```python
from build123d import *

# Parameters (mm, degrees)
SKETCH1_R           = 3.175
BOSS_EXTRUDE1_DEPTH = 20.6
SKETCH2_R           = 19.05
BOSS_EXTRUDE2_DEPTH = 1.6
BOSS_EXTRUDE3_DEPTH = 4.8
BOSS_EXTRUDE4_DEPTH = 51.2
SKETCH7_W           = 3.420526276
SKETCH7_H           = 1.112659396
CUT_EXTRUDE5_DEPTH  = 15
CUT_EXTRUDE6_REACH  = 58
SKETCH8_R           = 2.55
CUT_EXTRUDE7_DEPTH  = 17


with BuildPart() as part:
    # Sketch1 → Boss-Extrude1 (new body)
    with BuildSketch(Plane.XY):
        Circle(SKETCH1_R)
    extrude(amount=BOSS_EXTRUDE1_DEPTH)

    # Sketch2 → Boss-Extrude2 (add)
    with BuildSketch(Plane(origin=(0, 0, 0), x_dir=(-1, 0, 0), z_dir=(0, 0, -1))):
        Circle(SKETCH2_R)
    extrude(amount=-BOSS_EXTRUDE2_DEPTH)

    # Sketch3 → Boss-Extrude3 (add)
    with BuildSketch(Plane(origin=(0, 0, 0), x_dir=(-1, 0, 0), z_dir=(0, 0, -1))):
        with BuildLine():
            Line((23.6, -28.2), (-23.6, -28.2))
            ThreePointArc((-23.6, -28.2), (-26.852691193, -26.852691193), (-28.2, -23.6))
            Line((-28.2, -23.6), (-28.2, 23.6))
            ThreePointArc((-28.2, 23.6), (-26.852691193, 26.852691193), (-23.6, 28.2))
            Line((-23.6, 28.2), (23.6, 28.2))
            ThreePointArc((23.6, 28.2), (26.852691193, 26.852691193), (28.2, 23.6))
            Line((28.2, 23.6), (28.2, -23.6))
            ThreePointArc((28.2, -23.6), (26.852691193, -26.852691193), (23.6, -28.2))
        make_face()
    extrude(amount=BOSS_EXTRUDE3_DEPTH)

    # Sketch4 → Boss-Extrude4 (add)
    with BuildSketch(Plane(origin=(0, 0, -4.8), x_dir=(-1, 0, 0), z_dir=(0, 0, -1))):
        with BuildLine():
            Line((-18.57, 23.57), (-18.57, 25.7))
            ThreePointArc((-18.57, 25.7), (-17.837766953, 27.467766953), (-16.07, 28.2))
            Line((-16.07, 28.2), (16.07, 28.2))
            ThreePointArc((16.07, 28.2), (17.837766953, 27.467766953), (18.57, 25.7))
            Line((18.57, 25.7), (18.57, 23.57))
            ThreePointArc((18.57, 23.57), (20.034466094, 20.034466094), (23.57, 18.57))
            Line((23.57, 18.57), (25.7, 18.57))
            ThreePointArc((25.7, 18.57), (27.467766953, 17.837766953), (28.2, 16.07))
            Line((28.2, 16.07), (28.2, -16.07))
            ThreePointArc((28.2, -16.07), (27.467766953, -17.837766953), (25.7, -18.57))
            Line((25.7, -18.57), (23.57, -18.57))
            ThreePointArc((23.57, -18.57), (20.034466094, -20.034466094), (18.57, -23.57))
            Line((18.57, -23.57), (18.57, -25.7))
            ThreePointArc((18.57, -25.7), (17.837766953, -27.467766953), (16.07, -28.2))
            Line((16.07, -28.2), (-16.07, -28.2))
            ThreePointArc((-16.07, -28.2), (-17.837766953, -27.467766953), (-18.57, -25.7))
            Line((-18.57, -25.7), (-18.57, -23.57))
            ThreePointArc((-18.57, -23.57), (-20.034466094, -20.034466094), (-23.57, -18.57))
            Line((-23.57, -18.57), (-25.7, -18.57))
            ThreePointArc((-25.7, -18.57), (-27.467766953, -17.837766953), (-28.2, -16.07))
            Line((-28.2, -16.07), (-28.2, 16.07))
            ThreePointArc((-28.2, 16.07), (-27.467766953, 17.837766953), (-25.7, 18.57))
            Line((-25.7, 18.57), (-23.57, 18.57))
            ThreePointArc((-23.57, 18.57), (-20.034466094, 20.034466094), (-18.57, 23.57))
        make_face()
    extrude(amount=BOSS_EXTRUDE4_DEPTH)

    # Sketch7 → Cut-Extrude5 (cut)
    with BuildSketch(Plane.XY.offset(20.6)):
        with Locations((0, 3.231329698)):
            Rectangle(SKETCH7_W, SKETCH7_H)
    extrude(amount=-CUT_EXTRUDE5_DEPTH, mode=Mode.SUBTRACT)

    # Sketch8 → Cut-Extrude6 (cut, up to next)
    with BuildSketch(Plane.XY, mode=Mode.PRIVATE) as cut_extrude6_sk1:
        with Locations((-23.57, 23.57)):
            Circle(SKETCH8_R)
    cut_extrude6_tool1 = extrude(cut_extrude6_sk1.sketch, amount=-CUT_EXTRUDE6_REACH, mode=Mode.PRIVATE) & part.part
    add(cut_extrude6_tool1.solids().sort_by_distance((-23.57, 23.57, 0))[0], mode=Mode.SUBTRACT)
    # Sketch8 → Cut-Extrude6 (cut, up to next)
    with BuildSketch(Plane.XY, mode=Mode.PRIVATE) as cut_extrude6_sk2:
        with Locations((23.57, 23.57)):
            Circle(SKETCH8_R)
    cut_extrude6_tool2 = extrude(cut_extrude6_sk2.sketch, amount=-CUT_EXTRUDE6_REACH, mode=Mode.PRIVATE) & part.part
    add(cut_extrude6_tool2.solids().sort_by_distance((23.57, 23.57, 0))[0], mode=Mode.SUBTRACT)
    # Sketch8 → Cut-Extrude6 (cut, up to next)
    with BuildSketch(Plane.XY, mode=Mode.PRIVATE) as cut_extrude6_sk3:
        with Locations((23.57, -23.57)):
            Circle(SKETCH8_R)
    cut_extrude6_tool3 = extrude(cut_extrude6_sk3.sketch, amount=-CUT_EXTRUDE6_REACH, mode=Mode.PRIVATE) & part.part
    add(cut_extrude6_tool3.solids().sort_by_distance((23.57, -23.57, 0))[0], mode=Mode.SUBTRACT)
    # Sketch8 → Cut-Extrude6 (cut, up to next)
    with BuildSketch(Plane.XY, mode=Mode.PRIVATE) as cut_extrude6_sk4:
        with Locations((-23.57, -23.57)):
            Circle(SKETCH8_R)
    cut_extrude6_tool4 = extrude(cut_extrude6_sk4.sketch, amount=-CUT_EXTRUDE6_REACH, mode=Mode.PRIVATE) & part.part
    add(cut_extrude6_tool4.solids().sort_by_distance((-23.57, -23.57, 0))[0], mode=Mode.SUBTRACT)

    # Sketch9 → Cut-Extrude7 (cut, symmetric)
    with BuildSketch(Plane.XY.offset(-28)):
        with BuildLine():
            Line((18.57, 23.57), (18.57, 25.7))
            ThreePointArc((18.57, 25.7), (17.837766953, 27.467766953), (16.07, 28.2))
            Line((16.07, 28.2), (-16.07, 28.2))
            ThreePointArc((-16.07, 28.2), (-17.837766953, 27.467766953), (-18.57, 25.7))
            Line((-18.57, 25.7), (-18.57, 23.57))
            ThreePointArc((-18.57, 23.57), (-20.034466094, 20.034466094), (-23.57, 18.57))
            Line((-23.57, 18.57), (-25.7, 18.57))
            ThreePointArc((-25.7, 18.57), (-27.467766953, 17.837766953), (-28.2, 16.07))
            Line((-28.2, 16.07), (-28.2, -16.07))
            ThreePointArc((-28.2, -16.07), (-27.467766953, -17.837766953), (-25.7, -18.57))
            Line((-25.7, -18.57), (-23.57, -18.57))
            ThreePointArc((-23.57, -18.57), (-20.034466094, -20.034466094), (-18.57, -23.57))
            Line((-18.57, -23.57), (-18.57, -25.7))
            ThreePointArc((-18.57, -25.7), (-17.837766953, -27.467766953), (-16.07, -28.2))
            Line((-16.07, -28.2), (16.07, -28.2))
            ThreePointArc((16.07, -28.2), (17.837766953, -27.467766953), (18.57, -25.7))
            Line((18.57, -25.7), (18.57, -23.57))
            ThreePointArc((18.57, -23.57), (20.034466094, -20.034466094), (23.57, -18.57))
            Line((23.57, -18.57), (25.7, -18.57))
            ThreePointArc((25.7, -18.57), (27.467766953, -17.837766953), (28.2, -16.07))
            Line((28.2, -16.07), (28.2, 16.07))
            ThreePointArc((28.2, 16.07), (27.467766953, 17.837766953), (25.7, 18.57))
            Line((25.7, 18.57), (23.57, 18.57))
            ThreePointArc((23.57, 18.57), (20.034466094, 20.034466094), (18.57, 23.57))
        make_face()
        with BuildLine():
            Line((18.47, 23.57), (18.47, 25.7))
            ThreePointArc((18.47, 25.7), (17.767056275, 27.397056275), (16.07, 28.1))
            Line((16.07, 28.1), (-16.07, 28.1))
            ThreePointArc((-16.07, 28.1), (-17.767056275, 27.397056275), (-18.47, 25.7))
            Line((-18.47, 25.7), (-18.47, 23.57))
            ThreePointArc((-18.47, 23.57), (-19.963755416, 19.963755416), (-23.57, 18.47))
            Line((-23.57, 18.47), (-25.7, 18.47))
            ThreePointArc((-25.7, 18.47), (-27.397056275, 17.767056275), (-28.1, 16.07))
            Line((-28.1, 16.07), (-28.1, -16.07))
            ThreePointArc((-28.1, -16.07), (-27.397056275, -17.767056275), (-25.7, -18.47))
            Line((-25.7, -18.47), (-23.57, -18.47))
            ThreePointArc((-23.57, -18.47), (-19.963755416, -19.963755416), (-18.47, -23.57))
            Line((-18.47, -23.57), (-18.47, -25.7))
            ThreePointArc((-18.47, -25.7), (-17.767056275, -27.397056275), (-16.07, -28.1))
            Line((-16.07, -28.1), (16.07, -28.1))
            ThreePointArc((16.07, -28.1), (17.767056275, -27.397056275), (18.47, -25.7))
            Line((18.47, -25.7), (18.47, -23.57))
            ThreePointArc((18.47, -23.57), (19.963755416, -19.963755416), (23.57, -18.47))
            Line((23.57, -18.47), (25.7, -18.47))
            ThreePointArc((25.7, -18.47), (27.397056275, -17.767056275), (28.1, -16.07))
            Line((28.1, -16.07), (28.1, 16.07))
            ThreePointArc((28.1, 16.07), (27.397056275, 17.767056275), (25.7, 18.47))
            Line((25.7, 18.47), (23.57, 18.47))
            ThreePointArc((23.57, 18.47), (19.963755416, 19.963755416), (18.47, 23.57))
        make_face(mode=Mode.SUBTRACT)
    extrude(amount=CUT_EXTRUDE7_DEPTH, both=True, mode=Mode.SUBTRACT)


solid = part.part
```
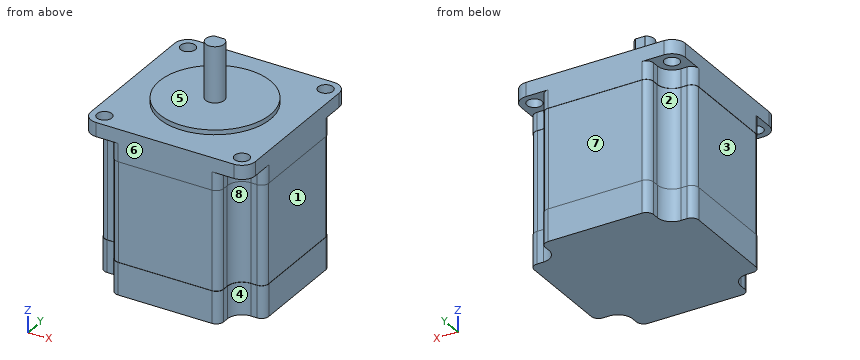
Can you work these out from the model? Positions are in its coordinate system, mm. Face numbers are marked on the shaded views. A direction names the side the tool comes from. Coordinates: 2 decimals unless noted, no trailing zeros. Write each loop counter-clockwise with the first axis right and the second up, starting at its lowest first coordinate (ties: lowest second). Pieces come first, ordered by that corner, then holes. Notation, with made-up numbers: M 1.25,-34.75 L 19.25,-34.75 A26 cw 19.25,4.25 Z; hole C -12.5,73.25 d4. An arc over 180 degrees is marked long. Write item = value, one per line. Start each with the question number.
Q1. If we section it at C-C, the plane y = 0: Write out the boundary of the cut face in (x, z) (3 decimals).
Q2. If we section it at A-A, the plane x = 0: Write out the boundary of the cut face in (y, z) (3 decimals).
Q3. If we section it at D-D, the plane z = -9: Write out the boundary of the cut face in (x, y).
Q4. If I drill on L1, parallel to Y at x = 23.57, z = -2.05; L2, parallel to Y at x = -23, z = -1, over which ranges is the centre line in solid material (lowest first)? Write a range as [from, to].
Q5. On a 3-axis mill with a long thin cutter (end or side, diameter ignored), from which of +Z, -Z, +X, -X, +Y, -Y can I reach the whole of each face in a straight line? I mean the marked faces 1, 2, 3 and 4. Say none if no direction works.
Q6. Thinking about a two-plate mould opening in Z: for the marked faces 5, 6, 7 and 8, which applies, released by +Z, released by -Z, zero draft, split by the parting line, or undercut?
Q7. I'm going to push flat-ended pins straight in: pin 1 (2 mm diameter, centred on x = -20, z = -43.5, fed in from +Y); pin 2 (1.1 mm diameter, centred on x = -24.5, z = -52, fed in from +Y); pin 3 (4.5 mm diameter, centred on x = 23.57, y = 23.57, fed in from +Z); pin 4 (2.5 mm diameter, centred on y = -24.5, z = -7.5, fed in from -X). Where does each tip first touch, or does it pass through?
Q8. If we section it at B-B, the plane z = -37: Write out the boundary of the cut face in (x, y).
Check sheet entries:
q1.outline = M -28.2,-56 L 28.2,-56 L 28.2,-45 L 28.1,-45 L 28.1,-11 L 28.2,-11 L 28.2,0 L 19.05,0 L 19.05,1.6 L 3.175,1.6 L 3.175,20.6 L -3.175,20.6 L -3.175,1.6 L -19.05,1.6 L -19.05,0 L -28.2,0 L -28.2,-11 L -28.1,-11 L -28.1,-45 L -28.2,-45 Z
q2.outline = M -28.2,-56 L 28.2,-56 L 28.2,-45 L 28.1,-45 L 28.1,-11 L 28.2,-11 L 28.2,0 L 19.05,0 L 19.05,1.6 L 3.175,1.6 L 3.175,5.6 L 2.675,5.6 L 2.675,20.6 L -3.175,20.6 L -3.175,1.6 L -19.05,1.6 L -19.05,0 L -28.2,0 L -28.2,-11 L -28.1,-11 L -28.1,-45 L -28.2,-45 Z
q3.outline = M -28.2,-16.07 A2.5 ccw -25.7,-18.57 L -23.57,-18.57 A5 cw -18.57,-23.57 L -18.57,-25.7 A2.5 ccw -16.07,-28.2 L 16.07,-28.2 A2.5 ccw 18.57,-25.7 L 18.57,-23.57 A5 cw 23.57,-18.57 L 25.7,-18.57 A2.5 ccw 28.2,-16.07 L 28.2,16.07 A2.5 ccw 25.7,18.57 L 23.57,18.57 A5 cw 18.57,23.57 L 18.57,25.7 A2.5 ccw 16.07,28.2 L -16.07,28.2 A2.5 ccw -18.57,25.7 L -18.57,23.57 A5 cw -23.57,18.57 L -25.7,18.57 A2.5 ccw -28.2,16.07 Z
q4.L1 = [-28.2, -26.12], [-21.02, 21.02], [26.12, 28.2]
q4.L2 = [-28.2, -26.06], [-21.08, 21.08], [26.06, 28.2]
q5.face_1 = +X, +Y, -Y
q5.face_2 = -X, +Y
q5.face_3 = -X, +Y, -Y
q5.face_4 = -Z, +X, -Y
q6.face_5 = released by +Z
q6.face_6 = zero draft
q6.face_7 = undercut
q6.face_8 = undercut
q7.pin_1 = 21.31
q7.pin_2 = 18.57
q7.pin_3 = through
q7.pin_4 = -18.58
q8.outline = M -28.1,-16.07 A2.4 ccw -25.7,-18.47 L -23.57,-18.47 A5.1 cw -18.47,-23.57 L -18.47,-25.7 A2.4 ccw -16.07,-28.1 L 16.07,-28.1 A2.4 ccw 18.47,-25.7 L 18.47,-23.57 A5.1 cw 23.57,-18.47 L 25.7,-18.47 A2.4 ccw 28.1,-16.07 L 28.1,16.07 A2.4 ccw 25.7,18.47 L 23.57,18.47 A5.1 cw 18.47,23.57 L 18.47,25.7 A2.4 ccw 16.07,28.1 L -16.07,28.1 A2.4 ccw -18.47,25.7 L -18.47,23.57 A5.1 cw -23.57,18.47 L -25.7,18.47 A2.4 ccw -28.1,16.07 Z
